Verification items for this drawing (mm, ordinates from the low corner). Give positions to 0.01 mm unless a question says otherwise; leave off trailing zeros. Order: outer loops, then holes, each group sorted by start corner. A loop starts at its lowest first (then second) coordinate and runs counter-clockwise, first axis right, second up. Notation, with made-up numbers: M 43.5,14 L 91.5,14 A10 ccw 91.5,28 Z; hole C 12.5,20 d1. An arc over 180 degrees is marked long. Return JSON: item names as keys, results as strings. Group by question number.
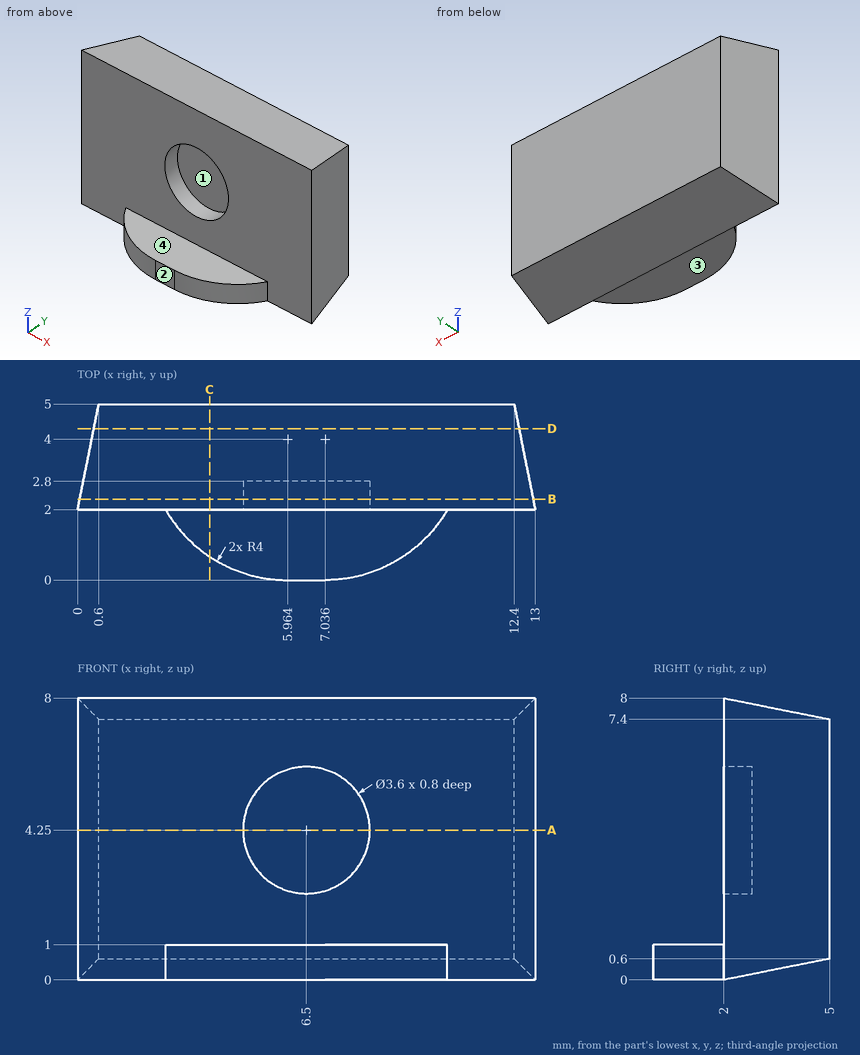
1) Release check for a two-part mould opening along Z. For the marked faces 1, 2, 3 and 4 record: released by +Z, released by -Z, zero draft, split by the parting line, or undercut.
2) Sectioned sample at C-C on x = 3.75. Record the boundary of the cut face in (y, z).
3) Material ranges on line 1 along Y through (x, z) = (2.25, 2.25); line 2 along X through (y, z) = (2.3, 4.25); line 3 along Y through (x, z) = (5.25, 4), recorded low to high.
4) Sectioned sample at B-B on y = 2.3. Record the boundary of the cut face in (x, z).
5) Sectioned sample at A-A on z = 4.25. Record the boundary of the cut face in (x, y).
6) Depth check by flat-ended pin: P1, Ø4, axis at x = 4.5, z = 5, coming from the -Y side; P2, Ø1, axis at x = 6, y = 3, coming from the -Z side; P3, Ø0.6, axis at x = 6, y = 1.5, coming from the +Z side. Enter the tip coordinate at first touch or a pass-through.
7) Sectioned sample at D-D on y = 4.3. Record the boundary of the cut face in (x, z).
Reply:
{
 "1": {"face 1": "undercut", "face 2": "zero draft", "face 3": "released by -Z", "face 4": "released by +Z"},
 "2": {"outline": "M 0.67,0 L 2,0 L 5,0.6 L 5,7.4 L 2,8 L 2,1 L 0.67,1 Z"},
 "3": {"line 1": "2 to 5", "line 2": "0.06 to 4.7, 8.3 to 12.94", "line 3": "2.8 to 5"},
 "4": {"outline": "M 0.06,0.06 L 12.94,0.06 L 12.94,7.94 L 0.06,7.94 Z; hole C 6.5,4.25 d3.6"},
 "5": {"outline": "M 0,2 L 4.7,2 L 4.7,2.8 L 8.3,2.8 L 8.3,2 L 13,2 L 12.4,5 L 0.6,5 Z"},
 "6": {"P1": "y = 2", "P2": "z = 0.1", "P3": "z = 1"},
 "7": {"outline": "M 0.46,0.46 L 12.54,0.46 L 12.54,7.54 L 0.46,7.54 Z"}
}
